```python
from build123d import *

# Parameters (mm, degrees)
F0_W     = 2.286
F0_H     = 38.1
F0_W_2   = 33.528
F0_R     = 6.35
F1_DEPTH = 2.286
F2_W     = 2.286
F2_H     = 38.1
F3_DEPTH = 73.914
F4_R     = 6.35
F5_DEPTH = 38.101


with BuildPart() as f1:
    # F0 (on Top) → F1 (new body)
    with BuildSketch(Plane.XY):
        with Locations((-14.750999, -1.450934)):
            Rectangle(F0_W, F0_H)
        with Locations((3.156001, -1.450934)):
            Rectangle(F0_W_2, F0_H)
        with Locations((3.156001, -1.450934)):
            Circle(F0_R, mode=Mode.SUBTRACT)
        with Locations((21.063001, -1.450934)):
            Rectangle(F0_W, F0_H)
    extrude(amount=F1_DEPTH)

    # F2 (on face) → F3 (join)
    with BuildSketch(Plane.XY.offset(2.286)):
        with Locations((-14.750999, -1.450934)):
            Rectangle(F2_W, F2_H)
        with Locations((21.063001, -1.450934)):
            Rectangle(F2_W, F2_H)
    extrude(amount=F3_DEPTH)

    # F4 (on face) → F5 (cut, through all)
    with BuildSketch(Plane.YZ.offset(22.206001)):
        with Locations((-1.450934, 57.15)):
            Circle(F4_R)
        with Locations((-1.450934, 38.1)):
            Circle(F4_R)
        with Locations((-1.450934, 19.05)):
            Circle(F4_R)
    extrude(amount=-F5_DEPTH, mode=Mode.SUBTRACT)


solid = f1.part
```
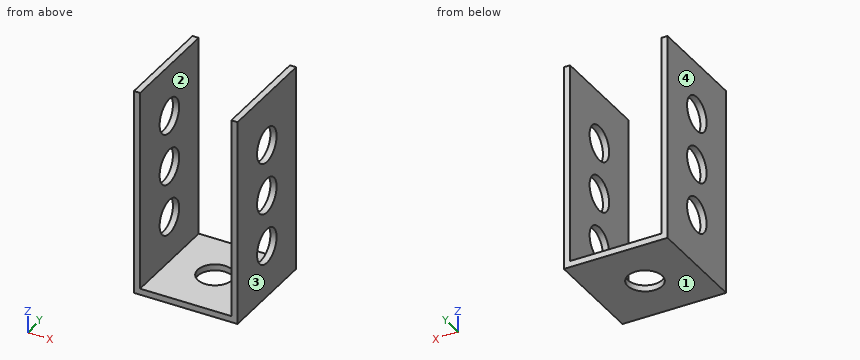
Verification items for the finished model (mm, model axes). Face numbers are marked on the shaded views. Coordinates: 2 decimals unless noted, no trailing zeros. Loops run counter-clockwise (first coordinate to the right, second up) from the corner with the lowest first, then second, coordinate; pieces in that order, holes last. Notation, with made-up numbers: (-10.5, -32) - (1.5, -32) arc R31 cw to (1.5, 4) - close; hole circle Ø2 at (-20, -29). An arc over 180 degrees is marked (long way). Answer as a JSON object with one key per item and string values.
(1) Cross-section at A-A, the plane z = 57.15. Record the boundary of the cut face in (x, y), then the cut area to 3 significant figures.
Response:
{"outline": "(-15.89, -20.5) - (-13.61, -20.5) - (-13.61, -7.8) - (-15.89, -7.8) - close; (-15.89, 4.9) - (-13.61, 4.9) - (-13.61, 17.6) - (-15.89, 17.6) - close; (19.92, -20.5) - (22.21, -20.5) - (22.21, -7.8) - (19.92, -7.8) - close; (19.92, 4.9) - (22.21, 4.9) - (22.21, 17.6) - (19.92, 17.6) - close", "area": "116 mm²"}
(2) Cross-section at B-B, the plane z = 28. Record the boundary of the cut face in (x, y), then the cut area to 3 significant figures.
Response:
{"outline": "(-15.89, -20.5) - (-13.61, -20.5) - (-13.61, 17.6) - (-15.89, 17.6) - close; (19.92, -20.5) - (22.21, -20.5) - (22.21, 17.6) - (19.92, 17.6) - close", "area": "174 mm²"}
(3) Go/stop test with flat-tipped pins: pin 1 Ø16.5 at (y, z) = (-1.45, 19.05) entering from -X; pin 2 Ø17 at (x, y) = (11, 4.5) entering from +Z. Record where each tip stops, or that it passes through.
Response:
{"pin 1": "stops at x = -15.89", "pin 2": "stops at z = 2.29"}
(4) Cross-section at D-D, the plane y = -13.5. Record the boundary of the cut face in (x, z), then the cut area to 3 significant figures.
Response:
{"outline": "(-15.89, 0) - (22.21, 0) - (22.21, 76.2) - (19.92, 76.2) - (19.92, 2.29) - (-13.61, 2.29) - (-13.61, 76.2) - (-15.89, 76.2) - close", "area": "425 mm²"}
(5) Cross-section at C-C, the plane x = 8. Record the boundary of the cut face in (y, z).
Response:
{"outline": "(-20.5, 0) - (-5.56, 0) - (-5.56, 2.29) - (-20.5, 2.29) - close; (2.65, 0) - (17.6, 0) - (17.6, 2.29) - (2.65, 2.29) - close"}
(6) Scan lines: line 1 along X through (y, z) = (14, 14.5); line 2 along Y through (x, z) = (-15, 38); line 3 along Z through (x, y) = (16.5, -15.5). Record each from-to range of solid material in increasing order.
Response:
{"line 1": "x = -15.89 to -13.61, 19.92 to 22.21", "line 2": "y = -20.5 to -7.8, 4.9 to 17.6", "line 3": "z = 0 to 2.29"}
(7) Mould release check, pull along X, two halves, no side actions. Record for the marked faces 1, 2, 3 and 4: pulls with the +X half, pulls with the -X half, needs draft (parallel to the pull), parting line crosses it, or undercut.
Response:
{"face 1": "needs draft", "face 2": "undercut", "face 3": "pulls with the +X half", "face 4": "pulls with the -X half"}
